from build123d import *

# Parameters (mm, degrees)
EXTRUDE_1_DEPTH     = 15
SKETCH_2_R          = 11
CUT_EXTRUDE_1_DEPTH = 51.0999002
SKETCH_3_R          = 13
CUT_EXTRUDE_2_DEPTH = 13
SKETCH_4_R          = 2.75
CUT_EXTRUDE_3_DEPTH = 51.0999002


with BuildPart() as part:
    # 草图1 → 凸台-拉伸1 (new body)
    with BuildSketch(Plane.XY):
        Polygon((29, 0), (-29, 0), (-29, 10), (-17, 10), (-17, 38), (17, 38), (17, 10), (29, 10), align=None)
    extrude(amount=EXTRUDE_1_DEPTH)

    # 草图2 → 切除-拉伸1 (cut, through all)
    with BuildSketch(Plane(origin=(0, 0, 0), x_dir=(-1, 0, 0), z_dir=(0, 0, -1))):
        with Locations((0, 20)):
            Circle(SKETCH_2_R)
    extrude(amount=-CUT_EXTRUDE_1_DEPTH, mode=Mode.SUBTRACT)

    # 草图3 → 切除-拉伸2 (cut)
    with BuildSketch(Plane(origin=(0, 0, 0), x_dir=(-1, 0, 0), z_dir=(0, 0, -1))):
        with Locations((0, 20)):
            Circle(SKETCH_3_R)
    extrude(amount=-CUT_EXTRUDE_2_DEPTH, mode=Mode.SUBTRACT)

    # 草图4 → 切除-拉伸3 (cut, through all)
    with BuildSketch(Plane.XZ):
        with Locations(Location((-23, 7.5, 0), (0, 0, 270))):
            Circle(SKETCH_4_R)
        with Locations((23, 7.5)):
            Circle(SKETCH_4_R)
    extrude(amount=-CUT_EXTRUDE_3_DEPTH, mode=Mode.SUBTRACT)


solid = part.part
Here's how the part is built. I have some questions about the finished solid (model axes, mm). A direction names the side the tool comes from. Round coordinates to 2 decimals unless told otherwise and drop trailing zeros. Loops run counter-clockwise (first coordinate to the right, second up) from the corner with the lowest first, then second, coordinate; pieces in that order, holes last.
1. If I drill on line 1 along Y through (x, z) = (0, 13.6); line 2 along Y through (x, z) = (-0.5, 9); line 3 along X through (y, z) = (2.5, 8), over which ranges is the centre line in solid material (lowest first)?
Answer list:
line 1: y = 0 to 9, 31 to 38
line 2: y = 0 to 7.01, 32.99 to 38
line 3: x = -29 to -25.7, -20.3 to 20.3, 25.7 to 29
2. If we section it at C-C on y = 20: Write out the boundary of the cut face in (x, z).
Answer list:
outline: (-17, 0) - (-13, 0) - (-13, 13) - (-11, 13) - (-11, 15) - (-17, 15) - close; (11, 13) - (13, 13) - (13, 0) - (17, 0) - (17, 15) - (11, 15) - close
3. We'd pull the mould along Y, two halves only. Please class faces 1 (the face through (17, 24, 7)), 2 (the face through (0, 38, 7)), 3 (the face through (1.69, 32.89, 6.41)): +Y half, -Y half, draft (parallel to the pull), parting line (faces both ways), or undercut.
Answer list:
face 1: draft
face 2: +Y half
face 3: undercut
4. If we section it at D-D on y = 5: Write out the boundary of the cut face in (x, z), plus the area to 3 significant figures.
Answer list:
outline: (-29, 0) - (29, 0) - (29, 15) - (-29, 15) - close; hole circle Ø5.5 at (-23, 7.5); hole circle Ø5.5 at (23, 7.5)
area: 822 mm2
5. If we section it at A-A on z = 7.5: Write out the boundary of the cut face in (x, y), plus the area to 3 significant figures.
Answer list:
outline: (-29, 0) - (-25.75, 0) - (-25.75, 10) - (-29, 10) - close; (-20.25, 0) - (20.25, 0) - (20.25, 10) - (17, 10) - (17, 38) - (-17, 38) - (-17, 10) - (-20.25, 10) - close; (25.75, 0) - (29, 0) - (29, 10) - (25.75, 10) - close; hole circle Ø26 at (0, 20)
area: 891 mm2
6. Which directions (+Z, -Z, +X, -X, +Y, -Y) give clear straight access to the entire face, cutting with the end or side of a thin tool? Please do faces 4 (the face through (29, 5, 7)), 5 (the face through (20, 10, 7)), 6 (the face through (0.4, 6.6, 0)), 7 (the face through (-17, 24, 7)), 8 (the face through (11, 23, 13)).
Answer list:
face 4: +Z, -Z, +X, +Y, -Y
face 5: +Z, -Z, +X, +Y
face 6: -Z, +X, -X, +Y, -Y
face 7: +Z, -Z, -X, +Y
face 8: -Z
7. If we section it at B-B on x = 23: Write out the boundary of the cut face in (y, z).
Answer list:
outline: (0, 0) - (10, 0) - (10, 4.75) - (0, 4.75) - close; (0, 10.25) - (10, 10.25) - (10, 15) - (0, 15) - close
8. For P1, Ø3.5, axis at x = 20.5, z = 6, coming from the +Y side; P2, Ø5, axis at y = 27.5, z = 12.5, coming from the +X side, each with a flat end and sliding along its axis, tell me the tip position at first contact or that it passes through.
Answer list:
P1: stops at y = 10
P2: stops at x = 17
